CAD build for the part. Positions are in the model's coordinates, mm. A direction names the side the tool comes from. Give positions to 0.01 mm unless a question says otherwise; leave off trailing zeros. Write each loop counter-clockwise with the first axis right and the second up, starting at its lowest first coordinate (ties: lowest second). Pieces come first, ordered by that corner, then holes. Notation, with made-up numbers: (-22, 81.5) -> (-2, 81.5) arc R12 ccw to (-2, 99.5) -> close; hole circle Ø2 at (17.5, 9). An arc over 180 degrees is marked (long way). Answer as a JSON object with one key per item and string values.
```python
from build123d import *

# Parameters (mm, degrees)
SZKIC3_R                    = 1.114790338
DODANIE_WYCI_GNI_CIE1_DEPTH = 5.5


with BuildPart() as part:
    # Szkic1 → Obrót2 (revolve)
    with BuildSketch(Plane.XY):
        Polygon((17, 0), (7, 0), (5.5, 0), (5.5, 2.829232786), (5.5, 4.829774456), (5.5, 7.237903332), (5.5, 9.045555295), (5.5, 11.058215628), (5.5, 12.5), (36, 12.5), (36, 9.045555295), (23, 9.045555295), (23, 8), (17, 8), align=None)
    revolve(axis=Axis((5.5, 12.5, 0), (1, 0, 0)))

    # Szkic3 → Dodanie-wyciągnięcie1 (add)
    with BuildSketch(Plane.ZY.offset(-5.5)):
        with Locations((-5.372694462, 4.139924233)):
            Circle(SZKIC3_R)
        with Locations((5.372694462, 4.139924233)):
            Circle(SZKIC3_R)
        with Locations((9.039596394, 8.371754652)):
            Circle(SZKIC3_R)
        with Locations((9.836490341, 13.9142738)):
            Circle(SZKIC3_R)
        with Locations((7.510368107, 19.00777101)):
            Circle(SZKIC3_R)
        with Locations((-2.799757064, 22.035096905)):
            Circle(SZKIC3_R)
        with Locations((-7.510368107, 19.00777101)):
            Circle(SZKIC3_R)
        with Locations((-9.836490341, 13.9142738)):
            Circle(SZKIC3_R)
        with Locations((-9.039596394, 8.371754652)):
            Circle(SZKIC3_R)
        with Locations((0, 2.5623588)):
            Circle(SZKIC3_R)
        with Locations((2.799757064, 22.035096905)):
            Circle(SZKIC3_R)
    extrude(amount=DODANIE_WYCI_GNI_CIE1_DEPTH)


solid = part.part
```
1) Pin check, flat tips, straight feed: pin 1 (10 mm diameter, centred on x = 18, z = 0, fed in from -Y); pin 2 (5 mm diameter, centred on x = 28.5, z = 6.5, fed in from +Y); pin 3 (1.5 mm diameter, centred on y = 21.5, z = 6, fed in from +X); pin 4 (5 mm diameter, centred on x = 17, z = -3.5, fed in from +Y). Stop position of each tip, or through.
Model answer:
{"pin 1": "stops at y = 0", "pin 2": "passes through", "pin 3": "stops at x = 17", "pin 4": "stops at y = 24.96"}
2) Slice it at B-B (y = 16.5). List the corners of the cut face in (x, z).
Model answer:
{"outline": "(5.5, -11.84) -> (17, -11.84) -> (17, -2.06) -> (23, -2.06) -> (23, 2.06) -> (17, 2.06) -> (17, 11.84) -> (5.5, 11.84) -> close"}
3) Slice it at D-D (z = -5). List the corners of the cut face in (x, y).
Model answer:
{"outline": "(0, 3.09) -> (5.5, 3.09) -> (5.5, 1.04) -> (17, 1.04) -> (17, 23.96) -> (5.5, 23.96) -> (5.5, 5.19) -> (0, 5.19) -> close"}
4) Slice it at A-A (z = 0). List the corners of the cut face in (x, y), then the cut area to 3 significant figures.
Model answer:
{"outline": "(0, 1.45) -> (5.5, 1.45) -> (5.5, 0) -> (17, 0) -> (17, 8) -> (23, 8) -> (23, 9.05) -> (36, 9.05) -> (36, 15.95) -> (23, 15.95) -> (23, 17) -> (17, 17) -> (17, 25) -> (5.5, 25) -> (5.5, 3.68) -> (0, 3.68) -> close", "area": "444 mm2"}
5) Slice it at C-C (x = 11.5). List the corners of the cut face in (y, z).
Model answer:
{"outline": "circle Ø25 at (12.5, 0)"}
6) 3-axis set-ups, long thin cutter, end or side, ignore diameter. For faces 1 (the cylindrical face through (2.788, 1.474, -0.242)), 2 (the flat face through (17, 12, 5)), 3 (the flat face through (0, 22, -3)): which of +Z, -Z, +X, -X, +Y, -Y reach the whole face in a straight line?
Model answer:
{"face 1": "-X", "face 2": "+X", "face 3": "+Z, -Z, -X, +Y, -Y"}
7) Mould opens along Z. For faces 4 (the flat face through (0, 3, 0)), 5 (the cylindrical face through (2.79, 23.14, 2.65)), 6 (the cylindrical face through (29.409, 15.241, 2.102)) say: released by +Z, released by -Z, zero draft, split by the parting line, or undercut.
Model answer:
{"face 4": "zero draft", "face 5": "undercut", "face 6": "split by the parting line"}
8) Wall check: probe 1 along Y at (x, z) = (20.5, 0); probe 2 along X at (y, z) = (17.75, -0.5); probe 3 along X at (y, z) = (13, -2). Give the ranges that are in metal, low to high.
Model answer:
{"probe 1": "y = 8 to 17", "probe 2": "x = 5.5 to 17", "probe 3": "x = 5.5 to 36"}
